```python
from build123d import *

# Parameters (mm, degrees)
BOSS_EXTRUDE1_DEPTH = 150
CHAMFER2_SIZE       = 0.4


with BuildPart() as part:
    # Sketch1 → Boss-Extrude1 (new body)
    with BuildSketch(Plane.XY):
        Polygon((5.95, 0.70711), (2.9, 0.70711), (2.9, 2.68877), (3.438098658, 2.759612032), (2.9, 3.60069), (1.9, 3.60069), (1.9, 0.70711), (-1.9, 0.70711), (-1.9, 3.60069), (-2.9, 3.60069), (-3.438098658, 2.759612032), (-2.9, 2.68877), (-2.9, 0.70711), (-5.95, 0.70711), (-5.24289, 0), (5.24289, 0), align=None)
    extrude(amount=BOSS_EXTRUDE1_DEPTH)

    # Chamfer2
    chamfer2_edges = [part.edges().sort_by_distance(p)[0] for p in [
        (5.596445, 0.353555, 0),
        (0, 0, 0),
        (-5.596445, 0.353555, 0),
        (-5.596445, 0.353555, 150),
        (0, 0, 150),
        (5.596445, 0.353555, 150),
    ]]
    chamfer(chamfer2_edges, length=CHAMFER2_SIZE)


solid = part.part
```
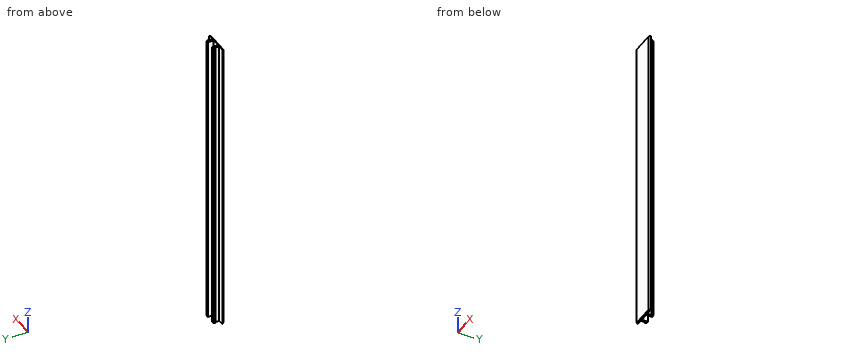
Source: CAD feature listing. Evaluate the final solid. Frame: model axes, mm. Give positions to 0.01 mm unless a question says otherwise; leave off trailing zeros. Order: outer loops, then holes, each group sorted by start corner. A loop starts at its lowest first (then second) coordinate and runs counter-clockwise, first axis right, second up.
(1) Material intervals for line 1 along Y through (x, z) = (3, 35.5); line 2 along X through (y, z) = (2.35, 22.5); line 3 along Y through (x, z) = (-1, 68), sorted ascending.
(2) Contact query for flat-ended pins moving along their axis: P1, Ø2, axis at y = 2.5, z = 68.5, coming from the -X side; P2, Ø2, axis at y = 1.5, z = 51, coming from the -X side; P3, Ø2, axis at y = 2, z = 99.5, coming from the +X side. Output: stop coordinate, or through.
(3) Section query B-B (z = 67). Return the cut outline in (x, y).
(4) Section query A-A (y = 1.25). Return the cut outline in (x, z).
Outcome:
1. line 1: y = 0 to 0.71, 2.7 to 3.44
1. line 2: x = -2.9 to -1.9, 1.9 to 2.9
1. line 3: y = 0 to 0.71
2. P1: stops at x = -3.44
2. P2: stops at x = -5.95
2. P3: stops at x = 3.44
3. outline: (-5.95, 0.71) - (-5.24, 0) - (5.24, 0) - (5.95, 0.71) - (2.9, 0.71) - (2.9, 2.69) - (3.44, 2.76) - (2.9, 3.6) - (1.9, 3.6) - (1.9, 0.71) - (-1.9, 0.71) - (-1.9, 3.6) - (-2.9, 3.6) - (-3.44, 2.76) - (-2.9, 2.69) - (-2.9, 0.71) - close
4. outline: (-2.9, 0) - (-1.9, 0) - (-1.9, 150) - (-2.9, 150) - close; (1.9, 0) - (2.9, 0) - (2.9, 150) - (1.9, 150) - close
